Verification items for the finished model (mm, model axes). A direction names the side the tool comes from. Round coordinates to 2 decimals unless told otherwise and drop trailing zeros. Write each loop counter-clockwise with the first axis right and the second up, starting at its lowest first coordinate (ties: lowest second). Pieces come first, ordered by that corner, then holes. Notation, with made-up numbers: M 61.25,2 L 86.25,2 A15 ccw 86.25,27 Z; hole C 80.25,79 d5. An arc over 180 degrees is marked long. One line per item, written item: value. Start each with the question number.
Item 1: Tool access check on faces 1 (the face through (161.85, 60.43, 2.35)), 2 (the face through (308.908, -84.464, 2.421)). Record the directions out of +Z, -Z, +X, -X, +Y, -Y that give a thin tool (end or side, any length) a straight path to the whole face; none if there is none.
Item 2: Section check A-A, the plane z = 3.3. Record the cut outline in (x, y), then the cut area to 3 significant figures.
Item 3: Section check B-B, the plane x = 115. Record the cut outline in (y, z).
Item 4: Gauge pin test, flat ends, axial feed: pin 1 (5 mm diameter, centred on x = -169, y = 27.5, fed in from -Z); pin 2 (1.5 mm diameter, centred on x = -183.5, z = 1.5, fed in from +Y). Record the tip position at first contact, or that the pin passes through.
Item 5: Section check C-C, the plane y = -180.5. Record the cut outline in (x, z).
Item 6: Draft check along X on faces 3 (the face through (432.99, -242.3, 2.35)), 4 (the face through (-161.85, 60.43, 2.35)), 5 (the face through (-41, -67, 4.775)). Enter one of: +X half, -X half, draft (parallel to the pull), parting line (faces both ways), or undercut.
Item 7: Thickness scan on probe 1 along X at (y, z) = (62, 4.45); probe 2 along X at (y, z) = (164.5, 2.7); probe 3 along X at (y, z) = (-202, 3.55). Record the ranges inside material, lowest first. Write a range as from..to.
from build123d import *

# Parameters (mm, degrees)
F1_DEPTH = 4.7752
F2_W     = 406.4
F2_H     = 4.7752
F3_DEPTH = 25.4
F4_W     = 406.4
F4_H     = 4.7752
F5_DEPTH = 25.4


with BuildPart() as f1:
    # F0 (on Top) → F1 (new body)
    with BuildSketch(Plane.XY):
        Polygon((423.6610569844, -250.6542817955), (0, 222.3534441402), (-423.6610569844, -250.6542817955), align=None)
    extrude(amount=F1_DEPTH)

    # F2 (on face) → F3 (join)
    with BuildSketch(Plane(origin=(110.5053208931, 98.9768210644, 0), x_dir=(-0.6671827669, 0.7448940566, 0), z_dir=(0.7448940566, 0.6671827669, 0))):
        with Locations((-266.1702409973, 2.3876)):
            Rectangle(F2_W, F2_H)
    extrude(amount=F3_DEPTH)

    # F4 (on face) → F5 (join)
    with BuildSketch(Plane(origin=(-110.5053208931, 98.9768210644, 0), x_dir=(-0.6671827669, -0.7448940566, 0), z_dir=(-0.7448940566, 0.6671827669, 0))):
        with Locations((266.1702409973, 2.3876)):
            Rectangle(F4_W, F4_H)
    extrude(amount=F5_DEPTH)


solid = f1.part
Response values:
1. face 1: +Z, -Z, +Y
1. face 2: +Z, -Z, +X, +Y
2. outline: M -442.58,-233.71 L -423.66,-250.65 L 423.66,-250.65 L 442.58,-233.71 L 171.44,69.02 L 152.52,52.07 L 0,222.35 L -152.52,52.07 L -171.44,69.02 Z
2. area: 221,000 mm2
3. outline: M -250.65,0 L 93.96,0 L 93.96,4.78 L -250.65,4.78 Z
4. pin 1: stops at z = 0
4. pin 2: stops at y = 56.39
5. outline: M -394.92,0 L 394.92,0 L 394.92,4.78 L -394.92,4.78 Z
6. face 3: +X half
6. face 4: undercut
6. face 5: draft
7. probe 1: x = -177.72..-163.6, -143.62..143.62, 163.6..177.72
7. probe 2: x = -51.82..51.82
7. probe 3: x = -414.18..414.18
